```python
from build123d import *

# Parameters (mm, degrees)
F0_R     = 18.36779
F1_DEPTH = 50.8
F2_R     = 3.616434
F2_W     = 6.643541
F2_H     = 6.132498


with BuildPart() as f1:
    # F0 (on Top) → F1 (new body)
    with BuildSketch(Plane.XY):
        Circle(F0_R)
    extrude(amount=F1_DEPTH)

    # F2 (on Right) → F3 (revolve, cut)
    with BuildSketch(Plane.YZ):
        with Locations((-19.738993, 41.785281)):
            Circle(F2_R)
        with Locations((-19.738992, 20.640921)):
            Rectangle(F2_W, F2_H)
    revolve(axis=Axis((0, 0, 23.766607), (0, 0, 1)), mode=Mode.SUBTRACT)


solid = f1.part
```
Verification items for the finished model (mm, model axes). A direction names the side the tool comes from. Give positions to 0.01 mm unless a question says otherwise; leave off trailing zeros. Order: outer loops, then holes, each group sorted by start corner. A loop starts at its lowest first (then second) coordinate and runs counter-clockwise, first axis right, second up. Notation, with made-up numbers: (16.5, -5.75) - (65.5, -5.75) arc R23 cw to (65.5, 17.25) - close; hole circle Ø2 at (76.5, 19). An arc over 180 degrees is marked (long way). Answer as CSV lines item,"result". Start each with the question number.
Item 1: Section check C-C, the plane z = 37.5. Record the boundary of the cut face in (x, y), plus the area to 3 significant figures.
Item 2: Material ranges on L1, parallel to Y at x = -0.5, z = 11; L2, parallel to Y at x = 7, z = 45.5; L3, parallel to X at y = 15.5, z = 38, recorded low to high.
Item 3: Mould release check, pull along Z, two halves, no side actions. Record for faces 1 (the face through (-2.39, 18.21, 8.66)), 2 (the face through (0, 0, 50.8)), 3 (the face through (-9, 14, 23.707)): released by +Z, released by -Z, zero draft, split by the parting line, or undercut.
Item 4: Section check A-A, the plane y = 0. Record the boundary of the cut face in (x, z), plus the area to 3 significant figures.
Item 5: Access from +Z, -Z, +X, -X, +Y, -Y to the whole of each face (thin tool, end or side, straight path). Record for faces 4 (the face through (-16.027, 3.559, 20.684)), 5 (the face through (-2.39, 18.21, 47.93)).
Item 6: Gauge pin test, flat ends, axial feed: pin 1 (8 mm diameter, centred on x = -13, z = 13.5, fed in from +Y); pin 2 (6 mm diameter, centred on y = -4.5, z = 24, fed in from +X); pin 3 (6 mm diameter, centred on x = 4.5, z = 35.5, fed in from -Y). Record the tip position at first contact, or that the pin passes through.
Filled in:
1,outline,"circle Ø36.74 at (0, 0)"
1,area,"1,060 mm^2"
2,L1,"-18.36 to 18.36"
2,L2,"-16.98 to 16.98"
2,L3,"-9.86 to 9.86"
3,face 1,"zero draft"
3,face 2,"released by +Z"
3,face 3,"undercut"
4,outline,"(-18.37, 0) - (18.37, 0) - (18.37, 17.57) - (16.42, 17.57) - (16.42, 23.71) - (18.37, 23.71) - (18.37, 38.44) arc R3.62 cw to (18.37, 45.13) - (18.37, 50.8) - (-18.37, 50.8) - (-18.37, 45.13) arc R3.62 cw to (-18.37, 38.44) - (-18.37, 23.71) - (-16.42, 23.71) - (-16.42, 17.57) - (-18.37, 17.57) - close"
4,area,"1,820 mm^2"
5,face 4,"none"
5,face 5,"+Z, -Z"
6,pin 1,"y = 16.01"
6,pin 2,"x = 18.31"
6,pin 3,"y = -18.31"
